The drawing under review shows one solid part. Ordinate dimensions are in mm from its lowest x, y, z. Round coordinates to 2 decimals unless told otherwise and drop trailing zeros. Order: outer loops, then holes, each group sorted by start corner. A loop starts at its lowest first (then second) coordinate and runs counter-clockwise, first axis right, second up.
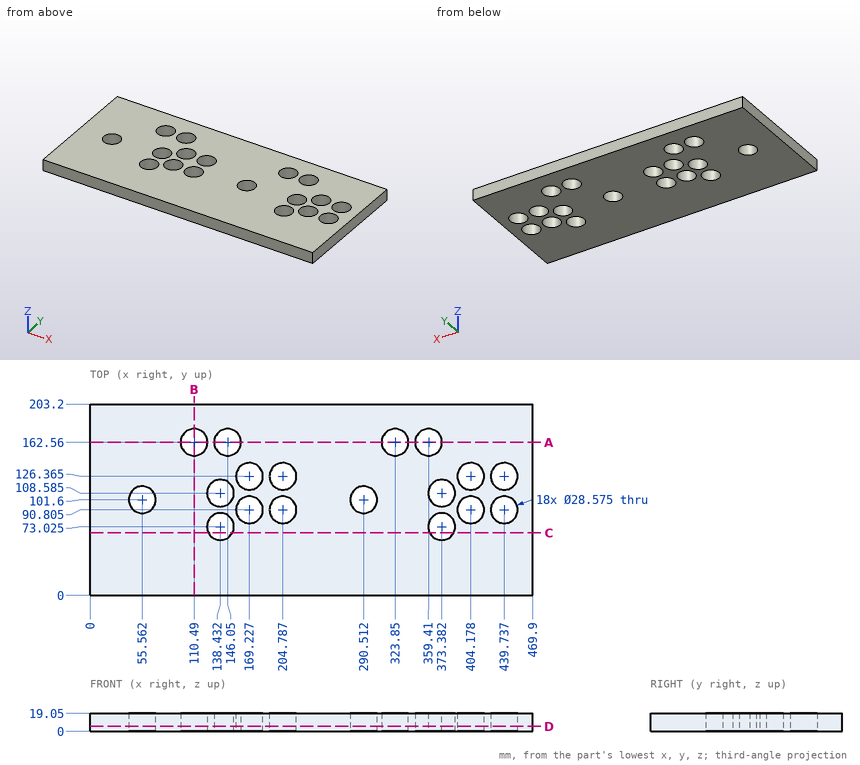
(1) We need section D-D (z = 5.25). Count the separate pieces of the cut face and the enclosed holes in it, and give its area (3 significant figures).
(2) To check wall thickness, follow L1, parallel to X at y = 72, z = 1; L2, parallel to Y at x = 391, z = 3 (1 decimal); L3, parallel to Y at x = 363, z = 14.5. State the ranges of each line that lie inside material, in increasing order.
(3) We need section B-B (x = 110.49). Give the boundary of the cut face in (y, z).
(4) We need section A-A (y = 162.56). Give the boundary of the cut face in (x, z).
(5) Clearance check with flat-ended pins moving along their axes: P1, Ø5, axis at x = 59.5, z = 7.5, coming from the -Y side; P2, Ø17, axis at x = 323.85, y = 162.56, coming from the +Z side. State where each tip first meets the part, or that it passes through.
(6) We need section C-C (y = 66.5). Give the boundary of the cut face in (x, z), and give its area (3 significant figures).
Verdict:
1. separate pieces: 1
1. enclosed holes: 18
1. area: 83,900 mm2
2. L1: x = 0 to 124.18, 152.68 to 359.13, 387.63 to 469.9
2. L2: y = 0 to 85.3, 96.3 to 120.8, 131.9 to 203.2
2. L3: y = 0 to 63.21, 82.84 to 98.77, 118.4 to 148.73, 176.39 to 203.2
3. outline: (0, 0) - (148.27, 0) - (148.27, 19.05) - (0, 19.05) - close; (176.85, 0) - (203.2, 0) - (203.2, 19.05) - (176.85, 19.05) - close
4. outline: (0, 0) - (96.2, 0) - (96.2, 19.05) - (0, 19.05) - close; (124.78, 0) - (131.76, 0) - (131.76, 19.05) - (124.78, 19.05) - close; (160.34, 0) - (309.56, 0) - (309.56, 19.05) - (160.34, 19.05) - close; (338.14, 0) - (345.12, 0) - (345.12, 19.05) - (338.14, 19.05) - close; (373.7, 0) - (469.9, 0) - (469.9, 19.05) - (373.7, 19.05) - close
5. P1: stops at y = 0
5. P2: passes through
6. outline: (0, 0) - (125.72, 0) - (125.72, 19.05) - (0, 19.05) - close; (151.14, 0) - (360.67, 0) - (360.67, 19.05) - (151.14, 19.05) - close; (386.09, 0) - (469.9, 0) - (469.9, 19.05) - (386.09, 19.05) - close
6. area: 7,980 mm2
